Source: CAD feature listing. Evaluate the final solid. Frame: model axes, mm. A direction names the side the tool comes from. Round coordinates to 2 decimals unless told otherwise and drop trailing zeros. Order: outer loops, then holes, each group sorted by start corner. A loop starts at its lowest first (then second) coordinate and runs counter-clockwise, first axis right, second up. Notation, with made-up numbers: (-4.75, -22) -> (44.25, -22) arc R13 ccw to (44.25, -7) -> close; hole circle Ø2 at (11.25, -26.75). An arc over 180 degrees is marked (long way). Write item = value, one per line. Start each with the question number.
(1) Contact query for flat-ended pins moving along their axis: pin 1 Ø1.5 at (x, z) = (-21, -36.5) entering from -Y; pin 2 Ø5 at (x, z) = (41, -34.5) entering from -Y; pin 3 Ø12 at (x, z) = (-7.5, -77.5) entering from -Y. Output: stop coordinate, or through.
(2) Cut plane C-C on x = 0. Return the cut outline in (y, z), then the cut area to 3 significant figures.
(3) Reachability of faces 3 (the face through (0.89, 11.44, -99.84)), 4 (the face through (0.89, 11.51, -100.06)) from +Z, -Z, +X, -X, +Y, -Y: full face, straight path, thin tool, end or side. Return the list, or none.
(4) Cut plane D-D on y = 33. Return the cut outline in (x, z).
(5) Cut plane A-A on y = 0. Return the cut outline in (x, z).
(6) Draft query along X for faces 1 (the face through (-8.259, -37.194, -24.25)), 2 (the face through (-8.309, -37.416, -24.25)). Return one class per face: released by +X, released by -X, zero draft, split by the parting line, or undercut.
(7) Ray query, line 1 (Y direction, x = 0, z = -13.5); line 2 (X direction, y = 21, z = -16); line 3 (Z direction, x = -32.5, y = -1). Return the intervals inside material, ascending.
(8) Cut plane B-B on z = -54. Return the cut outline in (x, y).
from build123d import *

# Parameters (mm, degrees)
SKETCH1_R           = 38.32733
BOSS_EXTRUDE2_DEPTH = 63.5
SKETCH2_R           = 38.32733
BOSS_EXTRUDE3_DEPTH = 127
SKETCH3_R           = 38.1
CUT_EXTRUDE1_DEPTH  = 128
SKETCH4_R           = 38.1
CUT_EXTRUDE2_DEPTH  = 63.5


with BuildPart() as part:
    # Sketch1 → Boss-Extrude2 (new body)
    with BuildSketch(Plane.XY):
        Circle(SKETCH1_R)
    extrude(amount=-BOSS_EXTRUDE2_DEPTH)

    # Sketch2 → Boss-Extrude3 (add)
    with BuildSketch(Plane(origin=(63.5, 0, 0), x_dir=(0, 0, -1), z_dir=(1, 0, 0))):
        with Locations((63.5, 0)):
            Circle(SKETCH2_R)
    extrude(amount=-BOSS_EXTRUDE3_DEPTH)

    # Sketch3 → Cut-Extrude1 (cut, through all)
    with BuildSketch(Plane(origin=(63.5, 0, 0), x_dir=(0, 0, -1), z_dir=(1, 0, 0))):
        with Locations((63.5, 0)):
            Circle(SKETCH3_R)
    extrude(amount=-CUT_EXTRUDE1_DEPTH, mode=Mode.SUBTRACT)

    # Sketch4 → Cut-Extrude2 (cut)
    with BuildSketch(Plane.XY):
        Circle(SKETCH4_R)
    extrude(amount=-CUT_EXTRUDE2_DEPTH, mode=Mode.SUBTRACT)


solid = part.part
Evaluation:
q1.pin_1 = -32.54
q1.pin_2 = -27.69
q1.pin_3 = -37.48
q2.outline = (-38.33, -63.5) arc R38.33 ccw to (38.33, -63.5) -> (38.33, 0) -> (38.1, 0) -> (38.1, -63.5) arc R38.1 cw to (-38.1, -63.5) -> (-38.1, 0) -> (-38.33, 0) -> close
q2.area = 56.2 mm^2
q3.face_3 = +X, -X
q3.face_4 = none
q4.outline = (-63.5, -82.99) -> (63.5, -82.99) -> (63.5, -82.54) -> (-63.5, -82.54) -> close; (-63.5, -44.46) -> (-19.04, -44.46) -> (-19.04, 0) -> (-19.49, 0) -> (-19.49, -44.01) -> (-63.5, -44.01) -> close; (19.04, -44.46) -> (63.5, -44.46) -> (63.5, -44.01) -> (19.49, -44.01) -> (19.49, 0) -> (19.04, 0) -> close
q5.outline = (-63.5, -101.83) -> (63.5, -101.83) -> (63.5, -101.6) -> (-63.5, -101.6) -> close; (-63.5, -25.4) -> (-38.1, -25.4) -> (-38.1, 0) -> (-38.33, 0) -> (-38.33, -25.17) -> (-63.5, -25.17) -> close; (38.1, -25.4) -> (63.5, -25.4) -> (63.5, -25.17) -> (38.33, -25.17) -> (38.33, 0) -> (38.1, 0) -> close
q6.face_1 = undercut
q6.face_2 = split by the parting line
q7.line_1 = -38.33 to -38.1, 38.1 to 38.33
q7.line_2 = -32.06 to -31.79, 31.79 to 32.06
q7.line_3 = -101.81 to -101.59
q8.outline = (-63.5, -37.13) -> (-9.5, -37.13) arc R38.33 ccw to (9.5, -37.13) -> (63.5, -37.13) -> (63.5, -36.9) -> (9.5, -36.9) arc R38.1 cw to (-9.5, -36.9) -> (-63.5, -36.9) -> close; (-63.5, 36.9) -> (-9.5, 36.9) arc R38.1 cw to (9.5, 36.9) -> (63.5, 36.9) -> (63.5, 37.13) -> (9.5, 37.13) arc R38.33 ccw to (-9.5, 37.13) -> (-63.5, 37.13) -> close
